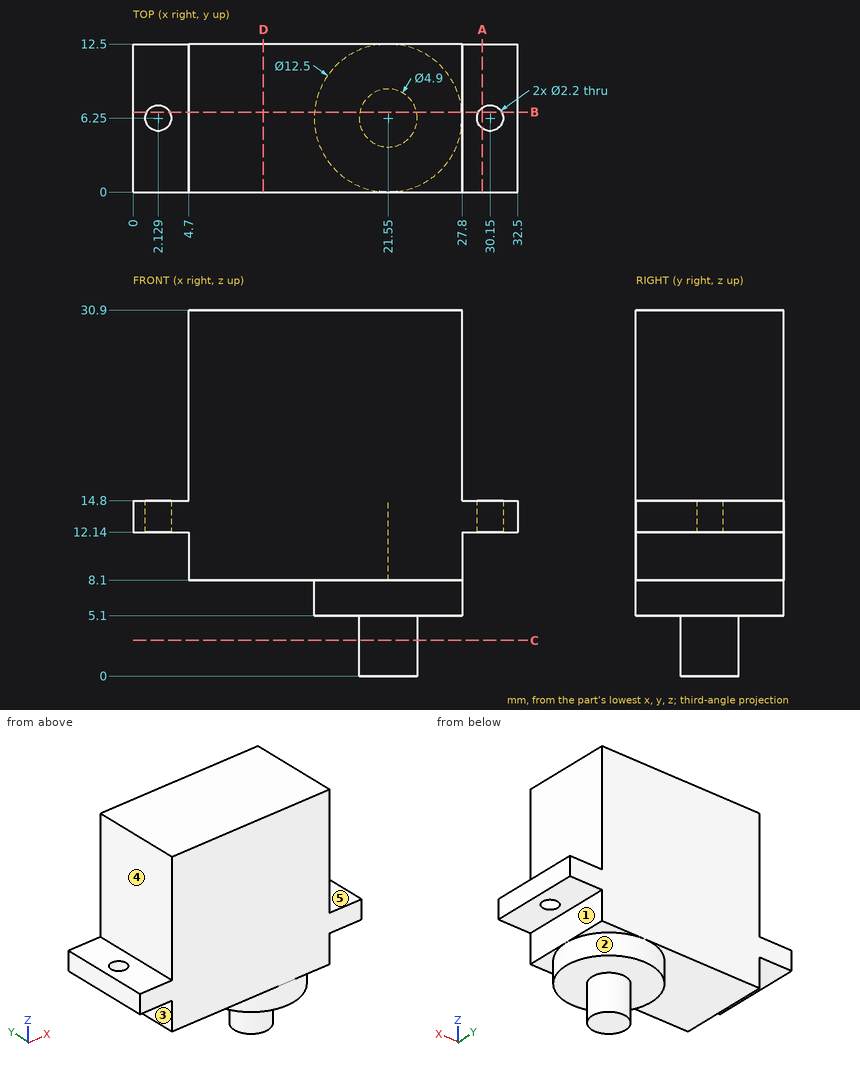
Part print with two shaded views. Sizes in mm from the minimum x, y, z corner. A direction names the side the tool comes from. Round coordinates to 2 decimals unless told otherwise and drop trailing zeros. Order: outer loops, then holes, each group sorted by start corner. A loop starts at its lowest first (then second) coordinate and runs counter-clockwise, first axis right, second up. Notation, with made-up numbers: M -8.75,-5 L 30.25,-5 A26 ccw 30.25,14 Z; hole C 20,-12 d4. An arc over 180 degrees is marked long. Use CSV: the item, a comma, the result in double quotes.
Item 1: Saw through at C-C (z = 3). List the corners of the cut face in (x, y).
Worked answers:
outline,"C 21.55,6.25 d4.9"
Item 2: Pin check, flat tips, straight feed: pin 1 (3 mm diameter, centred on x = 12.5, y = 3, fed in from -Z); pin 2 (3 mm diameter, centred on x = 26, y = 3.5, fed in from -Z); pin 3 (4 mm diameter, centred on x = 30, y = 7, fed in from +Z); pin 4 (5 mm diameter, centred on y = 3, z = 16.5, fed in from -X). Stop position of each tip, or through.
Worked answers:
pin 1,"z = 8.1"
pin 2,"z = 5.1"
pin 3,"z = 14.8"
pin 4,"x = 0"
Item 3: Saw through at A-A (x = 29.5). List the corners of the cut face in (y, z).
Worked answers:
outline,"M 0,12.14 L 5.36,12.14 L 5.36,14.8 L 0,14.8 Z; M 7.14,12.14 L 12.5,12.14 L 12.5,14.8 L 7.14,14.8 Z"
Item 4: Saw through at B-B (y = 6.75). State how many separate pieces and enclosed holes the cut face has, plus the area to 3 significant figures.
Worked answers:
separate pieces,"3"
enclosed holes,"0"
area,"603 mm²"
Item 5: Saw through at D-D (x = 11). List the corners of the cut face in (y, z).
Worked answers:
outline,"M 0,8.1 L 12.5,8.1 L 12.5,30.9 L 0,30.9 Z"
Item 6: Probe probe 1 along Y at (x, z) = (30.15, 13); probe 2 along X at (y, z) = (5.5, 13) (1 decimal); probe 3 along Z at (x, y) = (23.5, 2.75). List the from-to ranges inside material, lowest first.
Worked answers:
probe 1,"0 to 5.15, 7.35 to 12.5"
probe 2,"0 to 1.3, 2.9 to 29.3, 31 to 32.5"
probe 3,"5.1 to 30.9"
Item 7: Which spindle directions (+Z, -Z, +X, -X, +Y, -Y) get a long thin tool onto all of the face, cutting with end or side? Do the marked faces 1, 2, 3, 4 and 5. Say none if no direction does.
Worked answers:
face 1,"-Z, +X, +Y, -Y"
face 2,"-Z"
face 3,"-Z, -X, +Y, -Y"
face 4,"+Z, -X, +Y, -Y"
face 5,"+Z, +X, +Y, -Y"
